Input: part model. Units: mm. Frame: model coordinates. Face numbers are marked on the shaded views. Give positions to 0.01 mm unless a question says otherwise; leave off trailing zeros. Loops run counter-clockwise (first coordinate to the right, second up) from the corner with the lowest first, then second, coordinate; pieces in that order, holes last. Notation, with made-up numbers: M 14.25,43.5 L 67.25,43.5 A23 ccw 67.25,69.5 Z; hole C 80.25,-11 d7. An arc over 180 degrees is marked long. Answer as a JSON object with one key per item and string values. Group by question number.
1) First-contact query: P1, Ø1.9, axis at x = 0, y = 7, coming from the -Z side (1 decimal). Flat tip, straight axial feed; report the tip coordinate or a pass-through.
2) Draft query along Y for the marked faces 1, 2 and 3. Return one class per face: +Y half, -Y half, draft (parallel to the pull), parting line (faces both ways), or undercut.
3) Section query C-C on y = 7. Return loops of the section in (x, z), plus the area to 3 significant figures.
4) Section query A-A on x = 0. Return loops of the section in (y, z).
5) Section query D-D on z = 2. Return loops of the section in (x, y), plus the area to 3 significant figures.
6) Ray query, L1, parallel to Y at x = 0, z = 3.4; L2, parallel to Y at x = -7, z = 3.1; L3, parallel to X at y = -6.5, z = 4.4. Return the intervals inside material, ascending.
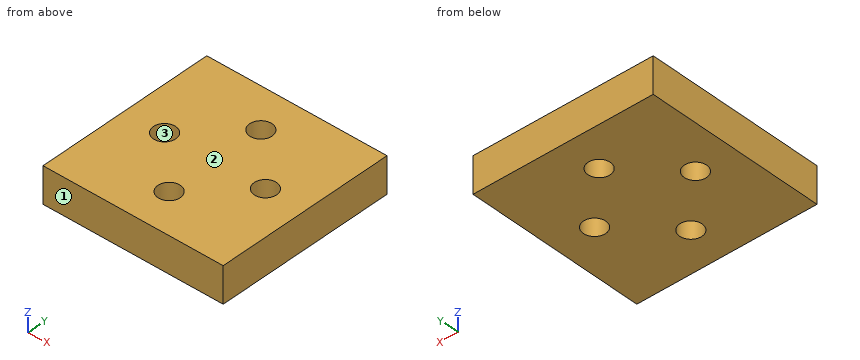
from build123d import *

# Parameters (mm, degrees)
SKETCH1_W           = 25
SKETCH1_H           = 25
SKETCH1_R           = 1.5
SKETCH1_R_2         = 1.551537049
BOSS_EXTRUDE1_DEPTH = 5
SKETCH2_R           = 1.55
BOSS_EXTRUDE2_DEPTH = 5


with BuildPart() as part:
    # Sketch1 → Boss-Extrude1 (new body)
    with BuildSketch(Plane.XY):
        Rectangle(SKETCH1_W, SKETCH1_H)
        Circle(SKETCH1_R, mode=Mode.SUBTRACT)
        with Locations((0, 7)):
            Circle(SKETCH1_R_2, mode=Mode.SUBTRACT)
        with Locations((7, 0)):
            Circle(SKETCH1_R_2, mode=Mode.SUBTRACT)
        with Locations((0, -7)):
            Circle(SKETCH1_R_2, mode=Mode.SUBTRACT)
        with Locations((-7, 0)):
            Circle(SKETCH1_R_2, mode=Mode.SUBTRACT)
    extrude(amount=BOSS_EXTRUDE1_DEPTH)

    # Sketch2 → Boss-Extrude2 (add)
    with BuildSketch(Plane.XY.offset(5)):
        Circle(SKETCH2_R)
    extrude(amount=-BOSS_EXTRUDE2_DEPTH)


solid = part.part
Output:
{
 "1": {"P1": "passes through"},
 "2": {"face 1": "-Y half", "face 2": "draft", "face 3": "undercut"},
 "3": {"outline": "M -12.5,0 L -1.55,0 L -1.55,5 L -12.5,5 Z; M 1.55,0 L 12.5,0 L 12.5,5 L 1.55,5 Z", "area": "109 mm^2"},
 "4": {"outline": "M -12.5,0 L -8.55,0 L -8.55,5 L -12.5,5 Z; M -5.45,0 L 5.45,0 L 5.45,5 L -5.45,5 Z; M 8.55,0 L 12.5,0 L 12.5,5 L 8.55,5 Z"},
 "5": {"outline": "M -12.5,-12.5 L 12.5,-12.5 L 12.5,12.5 L -12.5,12.5 Z; hole C -7,0 d3.1; hole C 0,-7 d3.1; hole C 0,7 d3.1; hole C 7,0 d3.1", "area": "595 mm^2"},
 "6": {"L1": "y = -12.5 to -8.55, -5.45 to 5.45, 8.55 to 12.5", "L2": "y = -12.5 to -1.55, 1.55 to 12.5", "L3": "x = -12.5 to -1.47, 1.47 to 12.5"}
}
